from build123d import *

# Parameters (mm, degrees)
SKETCH1_W           = 20
SKETCH1_H           = 40
SKETCH1_R           = 2.5
SKETCH1_R_2         = 4
BOSS_EXTRUDE1_DEPTH = 3
SKETCH2_R           = 5
CUT_EXTRUDE1_DEPTH  = 1.5
FILLET1_R           = 1.5


with BuildPart() as part:
    # Sketch1 → Boss-Extrude1 (new body)
    with BuildSketch(Plane.XY):
        Rectangle(SKETCH1_W, SKETCH1_H)
        with Locations((0, -10)):
            Circle(SKETCH1_R, mode=Mode.SUBTRACT)
        with Locations((0, 10)):
            Circle(SKETCH1_R, mode=Mode.SUBTRACT)
        Circle(SKETCH1_R_2, mode=Mode.SUBTRACT)
    extrude(amount=BOSS_EXTRUDE1_DEPTH)

    # Sketch2 → Cut-Extrude1 (cut)
    with BuildSketch(Plane.XY.offset(3)):
        with Locations((0, -10)):
            Circle(SKETCH2_R)
        with Locations((0, 10)):
            Circle(SKETCH2_R)
    extrude(amount=-CUT_EXTRUDE1_DEPTH, mode=Mode.SUBTRACT)

    # Fillet1
    fillet1_edges = [part.edges().sort_by_distance(p)[0] for p in [
        (-10, 20, 1.5),
        (10, 20, 1.5),
        (10, -20, 1.5),
        (-10, -20, 1.5),
    ]]
    fillet(fillet1_edges, radius=FILLET1_R)


solid = part.part
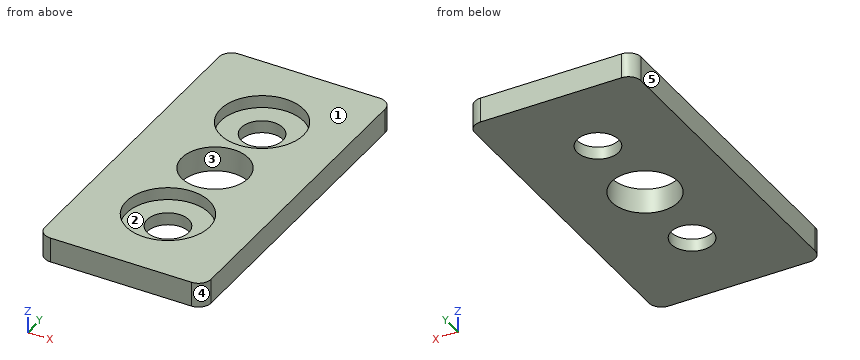
Here's how the part is built. I have some questions about the finished solid (model axes, mm). Face numbers are marked on the shaded views. A direction names the side the tool comes from. Round coordinates to 2 decimals unless told otherwise and drop trailing zeros. Write each loop counter-clockwise with the first axis right and the second up, starting at its lowest first coordinate (ties: lowest second). Pieces come first, ordered by that corner, then holes. Notation, with made-up numbers: (44.5, -38.75) -> (79.5, -38.75) arc R27 ccw to (79.5, -2.75) -> close; hole circle Ø3 at (-32.75, -14). An arc over 180 degrees is marked (long way). One line per item, written item: value.
1) If I drill on line 1 (Y direction, x = 0, z = 0.5); line 2 (Y direction, x = 0, z = 2.75); line 3 (Z direction, x = -0.5, y = 13), over which ranges is the centre line in solid material (lowest first)? Write a range as [from, to].
Filled sheet:
line 1: y = [-20, -12.5], [-7.5, -4], [4, 7.5], [12.5, 20]
line 2: y = [-20, -15], [-5, -4], [4, 5], [15, 20]
line 3: z = [0, 1.5]
2) Suppose I cut it at C-C on y = 10. List the corners of the cut face in (x, z) for me, plus the area to 3 significant figures.
Filled sheet:
outline: (-10, 0) -> (-2.5, 0) -> (-2.5, 1.5) -> (-5, 1.5) -> (-5, 3) -> (-10, 3) -> close; (2.5, 0) -> (10, 0) -> (10, 3) -> (5, 3) -> (5, 1.5) -> (2.5, 1.5) -> close
area: 37.5 mm2
3) Suppose I cut it at B-B on x = 0. List the corners of the cut face in (y, z) for me, plus the area to 3 significant figures.
Filled sheet:
outline: (-20, 0) -> (-12.5, 0) -> (-12.5, 1.5) -> (-15, 1.5) -> (-15, 3) -> (-20, 3) -> close; (-7.5, 0) -> (-4, 0) -> (-4, 3) -> (-5, 3) -> (-5, 1.5) -> (-7.5, 1.5) -> close; (4, 0) -> (7.5, 0) -> (7.5, 1.5) -> (5, 1.5) -> (5, 3) -> (4, 3) -> close; (12.5, 0) -> (20, 0) -> (20, 3) -> (15, 3) -> (15, 1.5) -> (12.5, 1.5) -> close
area: 51.0 mm2
4) We'd pull the mould along Y, two halves only. Please class the marked faces 3, 4 and 5: released by +Y, released by -Y, zero draft, split by the parting line, or undercut.
Filled sheet:
face 3: undercut
face 4: released by -Y
face 5: zero draft
5) For the marked faces 1 and 2, which set-ups out of +Z, -Z, +X, -X, +Y, -Y let a thin tool reach every point of the face, with its end or its side?
Filled sheet:
face 1: +Z, +X, -X, +Y, -Y
face 2: +Z
6) Suppose I cut it at A-A on y = 0. List the corners of the cut face in (x, z) for me, plus the area to 3 significant figures.
Filled sheet:
outline: (-10, 0) -> (-4, 0) -> (-4, 3) -> (-10, 3) -> close; (4, 0) -> (10, 0) -> (10, 3) -> (4, 3) -> close
area: 36.0 mm2
7) Suppose I cut it at D-D on y = -13. List the corners of the cut face in (x, z) for me.
Filled sheet:
outline: (-10, 0) -> (10, 0) -> (10, 3) -> (4, 3) -> (4, 1.5) -> (-4, 1.5) -> (-4, 3) -> (-10, 3) -> close
